CAD build for the part. Positions are in the model's coordinates, mm. A direction names the side the tool comes from. Give positions to 0.01 mm unless a question says otherwise; leave off trailing zeros. Loops run counter-clockwise (first coordinate to the right, second up) from the corner with the lowest first, then second, coordinate; pieces in that order, holes last.
Autodesk Inventor part; units mm, degrees
ref_plane "YZ Plane" through (0, 0, 0) normal (1, 0, 0) x (0, 1, 0)
ref_plane "XZ Plane" through (0, 0, 0) normal (0, 1, 0) x (-1, 0, 0)
ref_plane "XY Plane" through (0, 0, 0) normal (0, 0, 1) x (1, 0, 0)
sketch "Sketch1" plane through (0, 0, 0) normal (0, 1, 0) x (-1, 0, 0)
  line L0 (0, 0) -> (58, 0) construction
  line L1 (58, 0) -> (58, -49) construction
  line L2 (58, -49) -> (0, -49) construction
  line L3 (0, -49) -> (0, 0) construction
  circle A0 centre (58, -49) radius 1.6
  circle A1 centre (0, -49) radius 1.6
  circle A2 centre (58, 0) radius 1.6
  circle A3 centre (0, 0) radius 1.6
  line L4 (74, -24.5) -> (-16, -24.5) construction
  line L5 (29, -54.5) -> (29, 5.5) construction
  line L6 (69, -54.5) -> (-11, -54.5)
  line L7 (-16, -49.5) -> (-16, 0.5)
  line L8 (-11, 5.5) -> (69, 5.5)
  line L9 (74, 0.5) -> (74, -49.5)
  arc A4 (69, -54.5) -> (74, -49.5) centre (69, -49.5) ccw
  arc A5 (-16, -49.5) -> (-11, -54.5) centre (-11, -49.5) ccw
  arc A6 (-11, 5.5) -> (-16, 0.5) centre (-11, 0.5) ccw
  arc A7 (74, 0.5) -> (69, 5.5) centre (69, 0.5) ccw
  line L10 (-8, -49.5) -> (-6.5383, -49.5)
  line L11 (69, -46.5) -> (69, -2.5)
  line L12 (66, 0.5) -> (64.5383, 0.5)
  line L13 (-11, -2.5) -> (-11, -46.5)
  arc A8 (61.7362, -47.5714) -> (54.2638, -47.5714) centre (58, -49) ccw
  arc A9 (3.7362, -47.5714) -> (-3.7362, -47.5714) centre (0, -49) ccw
  arc A10 (-3.7362, -1.4286) -> (3.7362, -1.4286) centre (0, 0) ccw
  arc A11 (54.2638, -1.4286) -> (61.7362, -1.4286) centre (58, 0) ccw
  arc A12 (54.0314, -49.5) -> (61.9686, -49.5) centre (58, -49) ccw construction
  arc A13 (-3.9686, -49.5) -> (3.9686, -49.5) centre (0, -49) ccw construction
  arc A14 (3.9686, 0.5) -> (-3.9686, 0.5) centre (0, 0) ccw construction
  arc A15 (61.9686, 0.5) -> (54.0314, 0.5) centre (58, 0) ccw construction
  line L14 (64.5383, -49.5) -> (66, -49.5)
  line L15 (51.4617, 0.5) -> (6.5383, 0.5)
  line L16 (-6.5383, 0.5) -> (-8, 0.5)
  line L17 (6.5383, -49.5) -> (51.4617, -49.5)
  arc A16 (61.7362, -47.5714) -> (64.5383, -49.5) centre (64.5383, -46.5) ccw
  arc A17 (51.4617, -49.5) -> (54.2638, -47.5714) centre (51.4617, -46.5) ccw
  arc A18 (64.5383, 0.5) -> (61.7362, -1.4286) centre (64.5383, -2.5) ccw
  arc A19 (54.2638, -1.4286) -> (51.4617, 0.5) centre (51.4617, -2.5) ccw
  arc A20 (6.5383, 0.5) -> (3.7362, -1.4286) centre (6.5383, -2.5) ccw
  arc A21 (-3.7362, -1.4286) -> (-6.5383, 0.5) centre (-6.5383, -2.5) ccw
  arc A22 (-6.5383, -49.5) -> (-3.7362, -47.5714) centre (-6.5383, -46.5) ccw
  arc A23 (3.7362, -47.5714) -> (6.5383, -49.5) centre (6.5383, -46.5) ccw
  arc A24 (66, -49.5) -> (69, -46.5) centre (66, -46.5) ccw
  arc A25 (69, -2.5) -> (66, 0.5) centre (66, -2.5) ccw
  arc A26 (-8, 0.5) -> (-11, -2.5) centre (-8, -2.5) ccw
  arc A27 (-11, -46.5) -> (-8, -49.5) centre (-8, -46.5) ccw
  point P0 (29, -49)
  point P1 (0, -24.5)
  point P2 (58, -24.5)
  point P3 (29, 0)
  point P4 (29, -24.5)
  dimension "d0" = 3.2
  dimension "d1" = 58
  dimension "d2" = 49
  dimension "d3" = 5
  dimension "d4" = 90
  dimension "d5" = 60
  dimension "d6" = 5
  dimension "d7" = 8
  dimension "d8" = 5
  dimension "d9" = 5
  dimension "d10" = 5
  dimension "d11" = 3
extrude "Extrusion1" add sketch "Sketch1" along normal blind 3
equation "\"d8\" = d6"
equation "\"d9\" = d6"
equation "\"d10\" = d6"
properties part number "RemoteDisplayMount"
1. Pull direction X, two halves, no side cores. Call faces 3 (the face through (-4.858, 1.479, -48.985)), 4 (the face through (-28, 1, 5.5)), 5 (the face through (16, 1, -25)): released by +X, released by -X, zero draft, split by the parting line, or undercut.
Responses:
face 3: undercut
face 4: zero draft
face 5: released by +X
2. Drop flat-ended pins along their axis: pin 1 (3 mm diameter, centred on x = -58, z = -49, fed in from +Y); pin 2 (5 mm diameter, centred on x = 0, z = -49, fed in from +Y). Give the stop position or say it passes through.
Responses:
pin 1: passes through
pin 2: stops at y = 3
3. Saw through at C-C, the plane x = 0. List the corners of the cut face in (y, z), and give its area (3 significant figures).
Responses:
outline: (0, -54.5) - (3, -54.5) - (3, -50.6) - (0, -50.6) - close; (0, -47.4) - (3, -47.4) - (3, -45) - (0, -45) - close; (0, -4) - (3, -4) - (3, -1.6) - (0, -1.6) - close; (0, 1.6) - (3, 1.6) - (3, 5.5) - (0, 5.5) - close
area: 37.8 mm2
4. Saw through at A-A, the plane z = -10. List the corners of the cut face in (x, y).
Responses:
outline: (-74, 0) - (-69, 0) - (-69, 3) - (-74, 3) - close; (11, 0) - (16, 0) - (16, 3) - (11, 3) - close
5. Saw through at D-D, the plane y = 2.35. Count the separate pieces of the cut face and the enclosed holes in it, and give its area (3 significant figures).
Responses:
separate pieces: 1
enclosed holes: 5
area: 1,480 mm2
6. Tool access for faces 1 (the face through (-29, 1, 0.5)), 2 (the face through (-22, 3, 2)): list every direction of +Z, -Z, +X, -X, +Y, -Y with a clear straight run to the whole face (end or side of a thin tool).
Responses:
face 1: +Y, -Y
face 2: +Z, -Z, +X, -X, +Y
7. Probe line 1 along Z through (x, y) = (0, 1.95); line 2 along X through (y, z) = (2.5, -6); line 3 along Z through (x, y) = (-11, 1.85). List the from-to ranges inside material, lowest first.
Responses:
line 1: z = -54.5 to -50.6, -47.4 to -45, -4 to -1.6, 1.6 to 5.5
line 2: x = -74 to -69, 11 to 16
line 3: z = -54.5 to -49.5, 0.5 to 5.5
8. Saw through at B-B, the plane x = -25. List the corners of the cut face in (y, z), and give its area (3 significant figures).
Responses:
outline: (0, -54.5) - (3, -54.5) - (3, -49.5) - (0, -49.5) - close; (0, 0.5) - (3, 0.5) - (3, 5.5) - (0, 5.5) - close
area: 30.0 mm2
